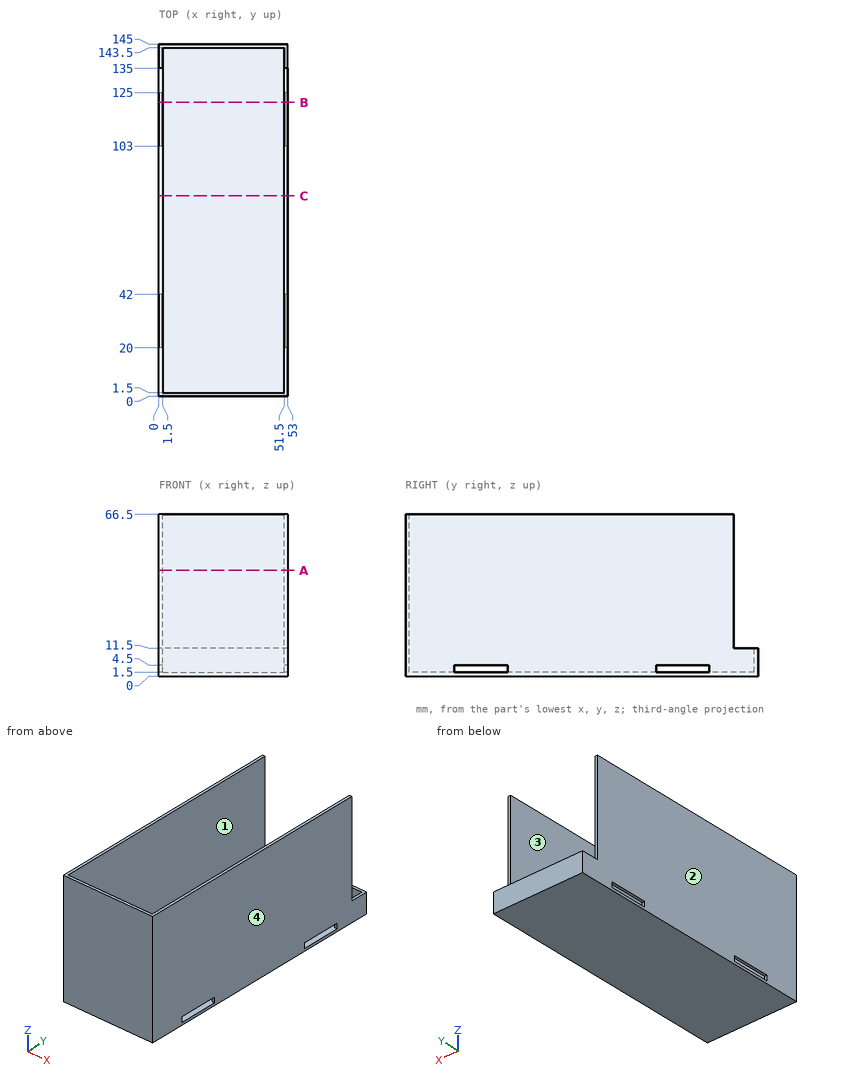
Part print with two shaded views. Sizes in mm from the minimum x, y, z corner. Round coordinates to 2 decimals unless told otherwise and drop trailing zeros. Order: outer loops, then holes, each group sorted by start corner. A loop starts at its lowest first (then second) coordinate and runs counter-clockwise, first axis right, second up.
(1) Drill centre lines: line 1 (X direction, y = 17.5, z = 38); line 2 (Y direction, x = 10, z = 10.5); line 3 (Z direction, x = 13.5, y = 22.5). Where is each one in solid material? Low to high.
(2) Band-saw the part on B-B (y = 121). List the corners of the cut face in (x, z), then the cut area to 4 significant figures.
(3) Band-saw the part on C-C (y = 82.5). List the corners of the cut face in (x, z), then the cut area to 4 significant figures.
(4) Pull direction X, two halves, no side cores. Call the marked faces 1, 2, 3 and 4: released by +X, released by -X, zero draft, split by the parting line, or undercut.
(5) Band-saw the part on A-A (z = 43.5). List the corners of the cut face in (x, y).
(6) Pin check, flat tips, straight feed: pin 1 (16 mm diameter, centred on x = 39.5, y = 44.5, fed in from +Z); pin 2 (1.5 mm diameter, centred on x = 29.5, z = 29.5, fed in from +Y). Stop position of each tip, or through.
Verdict:
1. line 1: x = 0 to 1.5, 51.5 to 53
1. line 2: y = 0 to 1.5, 143.5 to 145
1. line 3: z = 0 to 1.5
2. outline: (0, 0) - (53, 0) - (53, 1.5) - (0, 1.5) - close; (0, 4.5) - (1.5, 4.5) - (1.5, 66.5) - (0, 66.5) - close; (51.5, 4.5) - (53, 4.5) - (53, 66.5) - (51.5, 66.5) - close
2. area: 265.5 mm2
3. outline: (0, 0) - (53, 0) - (53, 66.5) - (51.5, 66.5) - (51.5, 1.5) - (1.5, 1.5) - (1.5, 66.5) - (0, 66.5) - close
3. area: 274.5 mm2
4. face 1: undercut
4. face 2: released by -X
4. face 3: undercut
4. face 4: released by +X
5. outline: (0, 0) - (53, 0) - (53, 135) - (51.5, 135) - (51.5, 1.5) - (1.5, 1.5) - (1.5, 135) - (0, 135) - close
6. pin 1: stops at z = 1.5
6. pin 2: stops at y = 1.5
